```python
from build123d import *

# Parameters (mm, degrees)
SKETCH1_R           = 5
BOSS_EXTRUDE1_DEPTH = 20
SKETCH2_R           = 8.6
BOSS_EXTRUDE2_DEPTH = 5
FILLET1_SIZE        = 2.5
FILLET1_SIZE_2      = 4
CUT_EXTRUDE1_DEPTH  = 4
FILLET2_R           = 0.5


with BuildPart() as part:
    # Sketch1 → Boss-Extrude1 (new body)
    with BuildSketch(Plane(origin=(0, 0, 0), x_dir=(1, 0, 0), z_dir=(0, 1, 0))):
        with Locations(Location((0, 0, 0), (0, 0, 270))):
            Circle(SKETCH1_R)
    extrude(amount=BOSS_EXTRUDE1_DEPTH)

    # Sketch2 → Boss-Extrude2 (add)
    with BuildSketch(Plane(origin=(0, 20, 0), x_dir=(1, 0, 0), z_dir=(0, 1, 0))):
        with Locations(Location((0, 0, 0), (0, 0, 270))):
            Circle(SKETCH2_R)
    extrude(amount=BOSS_EXTRUDE2_DEPTH)

    # Fillet1
    # an asymmetric fillet: 4, 2.5 mm, written as the material it takes off along each edge
    with BuildSketch(Plane(origin=(0, 25, 0), x_dir=(0, 0, 1), z_dir=(-1, 0, 0))) as fillet1_piece_1:
        with BuildLine():
            Bezier((8.6, -FILLET1_SIZE), (8.6, 0), (8.6 - FILLET1_SIZE_2, 0), weights=[1, 0.707106781, 1])
            Line((8.6 - FILLET1_SIZE_2, 0), (8.6, 0))
            Line((8.6, 0), (8.6, -FILLET1_SIZE))
        make_face()
    revolve(axis=Axis((0, 25, 0), (0, 1, 0)), mode=Mode.SUBTRACT)

    # Sketch3 → Cut-Extrude1 (cut)
    with BuildSketch(Plane(origin=(0, 25, 0), x_dir=(1, 0, 0), z_dir=(0, 1, 0))):
        Polygon((2.501014418, -2.520402127), (3.433239479, 0.905740958), (0.93222506, 3.426143085), (-2.501014418, 2.520402127), (-3.433239479, -0.905740958), (-0.93222506, -3.426143085), align=None)
    extrude(amount=-CUT_EXTRUDE1_DEPTH, mode=Mode.SUBTRACT)

    # Fillet2
    fillet2_edges = [part.edges().sort_by_distance(p)[0] for p in [
        (0, 20, -8.6),
    ]]
    fillet(fillet2_edges, radius=FILLET2_R)


solid = part.part
```
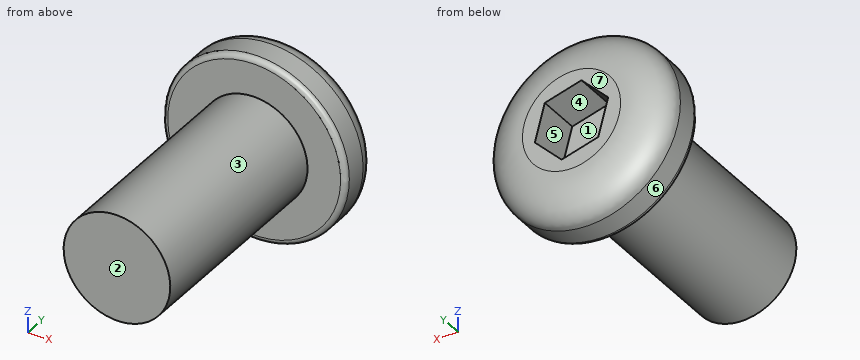
Check sheet for the modelled part. Datum: model origin and axes. Units: mm. Face numbers are marked on the shaded views. A direction names the side the tool comes from. Coordinates: 2 decimals unless noted, no trailing zeros. Loops run counter-clockwise (first coordinate to the right, second up) from the corner with the lowest first, then second, coordinate; pieces in that order, holes last.
1) Sectioned sample at A-A (y = 15.75). Record the boundary of the cut face in (x, z), and give its area (3 significant figures).
2) Material ranges on probe 1 along Y at (x, z) = (-2.25, -1.5); probe 2 along Z at (x, y) = (-1.75, 22.5); probe 3 along X at (y, z) = (12.5, -3.75), recorded low to high.
3) Access from +Z, -Z, +X, -X, +Y, -Y to the whole of each face (thin tool, end or side, straight path). Record for the marked faces 1, 2 and 3.
4) Gauge pin test, flat ends, axial feed: pin 1 (4 mm diameter, centred on x = 2.5, z = -3.5, fed in from -Y); pin 2 (3 mm diameter, centred on x = 4.5, y = 21.5, fed in from -Z); pin 3 (8 mm diameter, centred on y = 3.5, z = -4, fed in from +X); pin 4 (1.5 mm diameter, centred on y = 12, z = 0.5, fed in from -X). Record the tip position at first contact, or that the pin passes through.
5) Release check for a two-part mould opening along X. For the marked faces 4, 5, 6 and 7 record: released by +X, released by -X, zero draft, split by the parting line, or undercut.
Check sheet entries:
1. outline: circle Ø10 at (0, 0)
1. area: 78.5 mm2
2. probe 1: y = 0 to 21
2. probe 2: z = -8.42 to -2.72, 2.6 to 8.42
2. probe 3: x = -3.31 to 3.31
3. face 1: +Y
3. face 2: +Z, -Z, +X, -X, -Y
3. face 3: -Y
4. pin 1: stops at y = 0
4. pin 2: stops at z = -8.06
4. pin 3: stops at x = 5
4. pin 4: stops at x = -5
5. face 4: undercut
5. face 5: undercut
5. face 6: split by the parting line
5. face 7: zero draft
